```python
from build123d import *

# Parameters (mm, degrees)
F1_DEPTH = 3


with BuildPart() as f1:
    # F0 (on Front) → F1 (new body)
    with BuildSketch(Plane.XZ):
        Polygon((-75.109162, 1.415248), (-78.644696, 4.950781), (-76.495773, 7.099704), (-72.960239, 3.56417), (-64.50256, 12.021849), (-68.038094, 15.557383), (-65.887456, 17.705954), (-62.351922, 14.17042), (-53.894925, 22.627417), (-57.430459, 26.162951), (-55.280854, 28.312556), (-51.74532, 24.777022), (-43.288323, 33.234019), (-46.823857, 36.769553), (-44.674252, 38.919157), (-41.138718, 35.383623), (-32.681721, 43.84062), (-36.217255, 47.376154), (-34.067651, 49.525759), (-30.532117, 45.990225), (-22.07512, 54.447222), (-25.610654, 57.982756), (-23.461049, 60.132361), (-19.925515, 56.596827), (-11.468518, 65.053824), (-15.004052, 68.589358), (-12.854447, 70.738962), (-9.318913, 67.203429), (-0.861916, 75.660426), (-4.39745, 79.19596), (-2.247846, 81.345564), (1.287688, 77.81003), (10.635368, 87.15771), (11.155368, 87.67771), (11.155368, 88.67771), (11.155368, 89.62771), (12.635368, 89.62771), (12.635368, 103.301913), (12.155368, 102.821913), (-90.666545, 0), (-76.52441, 0), align=None)
    extrude(amount=F1_DEPTH)


solid = f1.part
```
Design review of the part built by this model. Coordinates are the model's own, in mm. A direction names the side the tool comes from. Coordinates: 2 decimals unless noted, no trailing zeros. Order: outer loops, then holes, each group sorted by start corner. A loop starts at its lowest first (then second) coordinate and runs counter-clockwise, first axis right, second up. Notation, with made-up numbers: M -25.5,-18.75 L 0.5,-18.75 A15 ccw 0.5,-3.75 Z; hole C 25,31.5 d4. An arc over 180 degrees is marked long. Answer as a JSON object with one key per item and string values. Group by question number.
1) Add section B-B, the plane z = 93.5. Write out the cut boundary in (x, y).
2) Mouldability with a two-part tool opening along Z and no side actions: class faces 3 (the flat face through (12.635, -1, 96)), 4 (the flat face through (-15.756, -1.479, 60.766)), 5 (the flat face through (-21.72, -1.48, 58.39)) as pulls with the +Z half, pulls with the -Z half, needs draft (parallel to the pull), parting line crosses it, or undercut.
3) Add section A-A, the plane x = -27. Write out the cut boundary in (y, z).
4) Wall thickness on L1, parallel to X at y = -1.25, z = 12; L2, parallel to Z at x = -55, y = -0.75; L3, parallel to Z at x = -12, y = -2.1: over which ranges is each line inside the solid? List them lowest first.
5) Tool access review of faces 1 (the flat face through (-53.54, -1.48, 26.57)), 2 (the flat face through (-58.18, -1.48, 18.34)): name each direction out of +Z, -Z, +X, -X, +Y, -Y from which nothing blocks a thin tool from reaching the whole face with its end or side.
6) For pin 1 (1.2 mm diameter, centred on x = 12, y = -1.5, fed in from -Z); pin 2 (1.6 mm diameter, centred on y = -1.5, z = 88.5, fed in from +X), all flat-tipped, find the tip position at first contact; note any pin that passes through.
Computed values:
{
 "1": {"outline": "M 2.83,-3 L 12.64,-3 L 12.64,0 L 2.83,0 Z"},
 "2": {"face 3": "needs draft", "face 4": "pulls with the -Z half", "face 5": "undercut"},
 "3": {"outline": "M -3,49.52 L 0,49.52 L 0,63.67 L -3,63.67 Z"},
 "4": {"L1": "x = -78.67 to -64.52", "L2": "z = 21.52 to 23.73, 28.03 to 35.67", "L3": "z = 64.52 to 65.59, 69.88 to 78.67"},
 "5": {"face 1": "+Y, -Y", "face 2": "-Z, +X, +Y, -Y"},
 "6": {"pin 1": "stops at z = 89.63", "pin 2": "stops at x = 11.16"}
}
